Can you work these out from the model? Positions are in its coordinate system, mm. Coordinates: 2 decimals unless noted, no trailing zeros. Order: outer loops, then holes, each group sorted by start corner. A loop starts at its lowest first (then second) coordinate and runs counter-clockwise, first axis right, second up. Notation, with made-up numbers: (15.25, 40) -> (25.25, 40) arc R13 cw to (25.25, 50) -> close; hole circle Ø11 at (21, 3). An arc over 180 degrees is marked (long way). Answer in a Markdown table with one row per item. Add a question column.
1. Imagine slicing it at D-D on z = 2.4. Write out the boundary of the cut face in (x, y).
2. Imagine slicing it at C-C on y = -2.15. Write out the boundary of the cut face in (x, z).
3. Imagine slicing it at A-A on z = 0. Write out the boundary of the cut face in (x, y).
4. If I drill on line 1 along Y through (x, z) = (23, -0.6); line 2 along Z through (x, y) = (14, 0.1); line 3 along Z through (x, y) = (5.25, -0.8), over which ranges is the centre line in solid material (lowest first)? Write a range as [from, to].
5. Will this pin go through, and if not, where does the flat tip stop? pin 1 (1.2 mm diameter, centred on y = 0, z = 0, fed in from -X).
6. Imagine slicing it at B-B on x = 16.75. Write out the boundary of the cut face in (y, z), plus the area to 3 significant figures.
from build123d import *

# Parameters (mm, degrees)
F0_R     = 1
F1_DEPTH = 30


with BuildPart() as f1:
    # F0 (on Right) → F1 (new body)
    with BuildSketch(Plane.YZ):
        Polygon((2.5, -1.443376), (2.5, 1.443376), (0, 2.886751), (-2.5, 1.443376), (-2.5, -1.443376), (0, -2.886751), align=None)
        Circle(F0_R, mode=Mode.SUBTRACT)
    extrude(amount=F1_DEPTH)


solid = f1.part
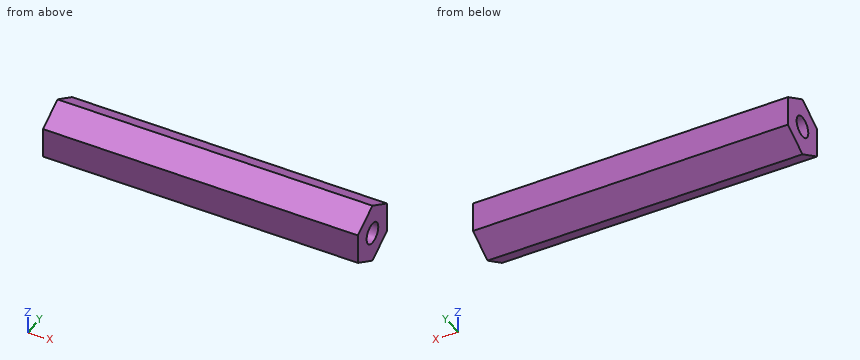
Answers follow:
| question | item | result |
|---|---|---|
| 1 | outline | (0, -0.84) -> (30, -0.84) -> (30, 0.84) -> (0, 0.84) -> close |
| 2 | outline | (0, -1.65) -> (30, -1.65) -> (30, 1.65) -> (0, 1.65) -> close |
| 3 | outline | (0, -2.5) -> (30, -2.5) -> (30, -1) -> (0, -1) -> close; (0, 1) -> (30, 1) -> (30, 2.5) -> (0, 2.5) -> close |
| 4 | line 1 | y = [-2.5, -0.8], [0.8, 2.5] |
| 4 | line 2 | z = [-2.83, -0.99], [0.99, 2.83] |
| 4 | line 3 | z = [-2.42, -0.6], [0.6, 2.42] |
| 5 | pin 1 | passes through |
| 6 | outline | (-2.5, -1.44) -> (0, -2.89) -> (2.5, -1.44) -> (2.5, 1.44) -> (0, 2.89) -> (-2.5, 1.44) -> close; hole circle Ø2 at (0, 0) |
| 6 | area | 18.5 mm² |
